from build123d import *

# Parameters (mm, degrees)
SKETCH1_W           = 160
SKETCH1_H           = 190
BOSS_EXTRUDE1_DEPTH = 18
SKETCH3_W           = 160
SKETCH3_H           = 14.25
CUT_EXTRUDE2_DEPTH  = 13.25
SKETCH4_W           = 160
SKETCH4_H           = 15.75
CUT_EXTRUDE3_DEPTH  = 13.25
SKETCH2_R           = 2.25
CUT_EXTRUDE1_DEPTH  = 126.495019822
SKETCH5_W           = 80
SKETCH5_H           = 131
CUT_EXTRUDE4_DEPTH  = 126.495019822
SKETCH6_W           = 85
SKETCH6_H           = 136
CUT_EXTRUDE5_DEPTH  = 2.5
SKETCH7_W           = 75
SKETCH7_H           = 12.75
CUT_EXTRUDE6_DEPTH  = 1.75
SKETCH8_W           = 88
SKETCH8_H           = 139
CUT_EXTRUDE7_DEPTH  = 1.25
SKETCH9_W           = 75
SKETCH9_H           = 14.25
CUT_EXTRUDE8_DEPTH  = 125.90221175
FILLET1_R           = 6
SKETCH10_W          = 15
SKETCH10_H          = 160
CUT_EXTRUDE9_DEPTH  = 13.25
CUT_EXTRUDE10_DEPTH = 126.495019822
FILLET2_R           = 10
FILLET3_R           = 5


with BuildPart() as part:
    # Sketch1 → Boss-Extrude1 (new body)
    with BuildSketch(Plane.XY):
        Rectangle(SKETCH1_W, SKETCH1_H)
    extrude(amount=BOSS_EXTRUDE1_DEPTH)

    # Sketch3 → Cut-Extrude2 (cut)
    with BuildSketch(Plane.XY.offset(18)):
        with Locations((0, 87.875)):
            Rectangle(SKETCH3_W, SKETCH3_H)
    extrude(amount=-CUT_EXTRUDE2_DEPTH, mode=Mode.SUBTRACT)

    # Sketch4 → Cut-Extrude3 (cut)
    with BuildSketch(Plane.XY.offset(18)):
        with Locations((0, -87.125)):
            Rectangle(SKETCH4_W, SKETCH4_H)
    extrude(amount=-CUT_EXTRUDE3_DEPTH, mode=Mode.SUBTRACT)

    # Sketch2 → Cut-Extrude1 (cut, through all)
    with BuildSketch(Plane(origin=(0, 0, 0), x_dir=(-1, 0, 0), z_dir=(0, 0, -1))):
        with Locations((-67.5, 88.5)):
            Circle(SKETCH2_R)
        with Locations((67.5, 88.5)):
            Circle(SKETCH2_R)
        with Locations((-72.5, -88.5)):
            Circle(SKETCH2_R)
        with Locations((72.5, -88.5)):
            Circle(SKETCH2_R)
    extrude(amount=-CUT_EXTRUDE1_DEPTH, mode=Mode.SUBTRACT)

    # Sketch5 → Cut-Extrude4 (cut, through all)
    with BuildSketch(Plane.XY.offset(18)):
        Rectangle(SKETCH5_W, SKETCH5_H)
    extrude(amount=-CUT_EXTRUDE4_DEPTH, mode=Mode.SUBTRACT)

    # Sketch6 → Cut-Extrude5 (cut)
    with BuildSketch(Plane.XY.offset(18)):
        Rectangle(SKETCH6_W, SKETCH6_H)
    extrude(amount=-CUT_EXTRUDE5_DEPTH, mode=Mode.SUBTRACT)

    # Sketch7 → Cut-Extrude6 (cut)
    with BuildSketch(Plane.XY.offset(18)):
        with Locations((0, 74.375)):
            Rectangle(SKETCH7_W, SKETCH7_H)
    extrude(amount=-CUT_EXTRUDE6_DEPTH, mode=Mode.SUBTRACT)

    # Sketch8 → Cut-Extrude7 (cut)
    with BuildSketch(Plane.XY.offset(18)):
        Rectangle(SKETCH8_W, SKETCH8_H)
    extrude(amount=-CUT_EXTRUDE7_DEPTH, mode=Mode.SUBTRACT)

    # Sketch9 → Cut-Extrude8 (cut, through all)
    with BuildSketch(Plane.XY.offset(4.75)):
        with Locations((0, 87.875)):
            Rectangle(SKETCH9_W, SKETCH9_H)
    extrude(amount=-CUT_EXTRUDE8_DEPTH, mode=Mode.SUBTRACT)

    # Fillet1
    fillet1_edges = [part.edges().sort_by_distance(p)[0] for p in [
        (0, 80.75, 16.25),
    ]]
    fillet(fillet1_edges, radius=FILLET1_R)

    # Sketch10 → Cut-Extrude9 (cut)
    with BuildSketch(Plane.XY.offset(18)):
        with Locations((72.5, 0.75)):
            Rectangle(SKETCH10_W, SKETCH10_H)
        with Locations((-72.5, 0.75)):
            Rectangle(SKETCH10_W, SKETCH10_H)
    extrude(amount=-CUT_EXTRUDE9_DEPTH, mode=Mode.SUBTRACT)

    # Sketch11 → Cut-Extrude10 (cut, through all)
    with BuildSketch(Plane(origin=(0, 0, 0), x_dir=(-1, 0, 0), z_dir=(0, 0, -1))):
        with BuildLine():
            Line((-74.75, -91), (-74.75, -86))
            ThreePointArc((-74.75, -86), (-72.5, -83.75), (-70.25, -86))
            Line((-70.25, -86), (-70.25, -91))
            ThreePointArc((-70.25, -91), (-72.5, -93.25), (-74.75, -91))
        make_face()
        with BuildLine():
            Line((70.25, -91), (70.25, -86))
            ThreePointArc((70.25, -86), (72.5, -83.75), (74.75, -86))
            Line((74.75, -86), (74.75, -91))
            ThreePointArc((74.75, -91), (72.5, -93.25), (70.25, -91))
        make_face()
    extrude(amount=-CUT_EXTRUDE10_DEPTH, mode=Mode.SUBTRACT)

    # Fillet2
    fillet2_edges = [part.edges().sort_by_distance(p)[0] for p in [
        (65, 80.75, 11.375),
        (65, -79.25, 11.375),
        (-65, -79.25, 11.375),
        (-65, 80.75, 11.375),
    ]]
    fillet(fillet2_edges, radius=FILLET2_R)

    # Fillet3
    fillet3_edges = [part.edges().sort_by_distance(p)[0] for p in [
        (-80, 95, 2.375),
        (80, 95, 2.375),
        (80, -95, 2.375),
        (-80, -95, 2.375),
    ]]
    fillet(fillet3_edges, radius=FILLET3_R)


solid = part.part
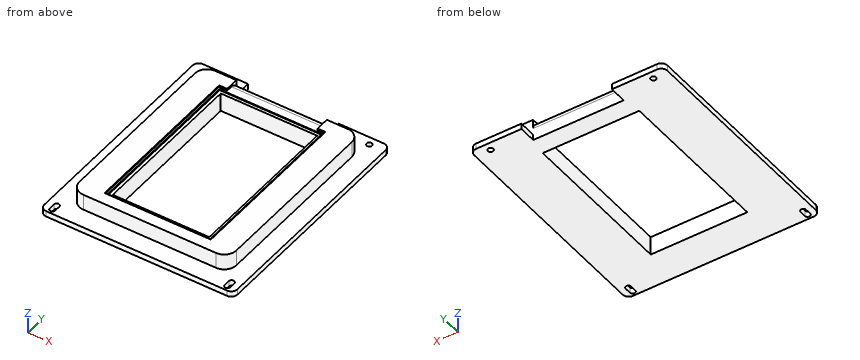
Design review of the part built by this model. Coordinates are the model's own, in mm. Coordinates: 2 decimals unless noted, no trailing zeros. Loops run counter-clockwise (first coordinate to the right, second up) from the corner with the lowest first, then second, coordinate; pieces in that order, holes last. Notation, with made-up numbers: (-31, 18.25) -> (27, 18.25) arc R26 cw to (27, 49.25) -> close; hole circle Ø1 at (0, 0.5). An arc over 180 degrees is marked (long way). Use a Markdown table: item, result. Add a question column.
Item 1: Clearance check with flat-ended pins moving along their axes: P1, Ø10, axis at y = 26, z = 14.5, coming from the -X side; P2, Ø0.6, axis at y = 33.5, z = 17.5, coming from the +X side; P3, Ø0.6, axis at x = 5, z = 17.5, coming from the +Y side. State where each tip first meets the part, or that it passes through.
Item 2: We need section C-C, the plane z = 2.25. Write out the cut boundary in (x, y), and give its area (3 significant figures).
Item 3: We need section B-B, the plane y = -44. Write out the cut boundary in (x, z).
Item 4: Wall thickness on L1, parallel to X at y = 28, z = 9.5; L2, parallel to X at y = 41.5, z = 3; L3, parallel to Y at x = -67.5, z = 1.15: over which ranges is each line inside the solid? List them lowest first. Write a range as from..to.
Item 5: We need section A-A, the plane x = 1.5. Write out the cut boundary in (y, z), and give its area (3 significant figures).
Item 6: We need section D-D, the plane z = 13. Write out the cut boundary in (x, y).
Numbers:
| question | item | result |
|---|---|---|
| 1 | P1 | stops at x = -65 |
| 1 | P2 | stops at x = 65 |
| 1 | P3 | stops at y = -69.5 |
| 2 | outline | (-80, -90) arc R5 ccw to (-75, -95) -> (75, -95) arc R5 ccw to (80, -90) -> (80, 90) arc R5 ccw to (75, 95) -> (37.5, 95) -> (37.5, 80.75) -> (-37.5, 80.75) -> (-37.5, 95) -> (-75, 95) arc R5 ccw to (-80, 90) -> close; hole (-74.75, -91) arc R2.25 ccw to (-70.25, -91) -> (-70.25, -86) arc R2.25 ccw to (-74.75, -86) -> close; hole circle Ø4.5 at (-67.5, 88.5); hole (-40, -65.5) -> (40, -65.5) -> (40, 65.5) -> (-40, 65.5) -> close; hole circle Ø4.5 at (67.5, 88.5); hole (70.25, -91) arc R2.25 ccw to (74.75, -91) -> (74.75, -86) arc R2.25 ccw to (70.25, -86) -> close |
| 2 | area | 18,700 mm^2 |
| 3 | outline | (-80, 0) -> (-40, 0) -> (-40, 15.5) -> (-42.5, 15.5) -> (-42.5, 16.75) -> (-44, 16.75) -> (-44, 18) -> (-65, 18) -> (-65, 4.75) -> (-80, 4.75) -> close; (40, 0) -> (80, 0) -> (80, 4.75) -> (65, 4.75) -> (65, 18) -> (44, 18) -> (44, 16.75) -> (42.5, 16.75) -> (42.5, 15.5) -> (40, 15.5) -> close |
| 4 | L1 | x = -65..-40, 40..65 |
| 4 | L2 | x = -80..-40, 40..80 |
| 4 | L3 | y = -95..86.25, 90.75..95 |
| 5 | outline | (-95, 0) -> (-65.5, 0) -> (-65.5, 15.5) -> (-68, 15.5) -> (-68, 16.75) -> (-69.5, 16.75) -> (-69.5, 18) -> (-79.25, 18) -> (-79.25, 4.75) -> (-95, 4.75) -> close; (65.5, 0) -> (80.75, 0) -> (80.75, 10.25) arc R6 ccw to (74.75, 16.25) -> (68, 16.25) -> (68, 15.5) -> (65.5, 15.5) -> close |
| 5 | area | 552 mm^2 |
| 6 | outline | (-65, -69.25) arc R10 ccw to (-55, -79.25) -> (55, -79.25) arc R10 ccw to (65, -69.25) -> (65, 70.75) arc R10 ccw to (55, 80.75) -> (37.5, 80.75) -> (37.5, 80.08) -> (-37.5, 80.08) -> (-37.5, 80.75) -> (-55, 80.75) arc R10 ccw to (-65, 70.75) -> close; hole (-40, -65.5) -> (40, -65.5) -> (40, 65.5) -> (-40, 65.5) -> close |
